from build123d import *

# Parameters (mm, degrees)
ESBO_O2_R                = 1.75
CORTE_EXTRUS_O1_DEPTH    = 6
ESBO_O3_R                = 4.25
CORTE_EXTRUS_O2_DEPTH    = 43.649736224
PADR_OCIRCULAR1_COUNT    = 4
CHANFRO1_SIZE            = 2
ESBO_O4_R                = 2
CORTE_EXTRUS_O3_DEPTH    = 46.639894829
PADR_OCIRCULAR2_COUNT    = 4
CHANFRO3_SIZE            = 2
RESSALTO_EXTRUS_O2_START = 2
ESBO_O5_R                = 12
ESBO_O5_R_2              = 1.75
RESSALTO_EXTRUS_O2_DEPTH = 2


with BuildPart() as part:
    # Esboço1 → Revolução1 (revolve)
    with BuildSketch(Plane.XY, mode=Mode.PRIVATE) as revolu_o1_sk:
        Polygon((0, 0), (0, 25), (27, 25), (27, 19), (12, 19), (12, 0), align=None)
    revolve(revolu_o1_sk.sketch.rotate(Axis((0, 0, 0), (0, 1, 0)), 90), axis=Axis((0, 0, 0), (0, 1, 0)))

    # Esboço2 → Corte-extrusão1 (cut)
    with BuildSketch(Plane.XZ):
        with Locations(Location((0, 7, 0), (0, 0, 270))):
            Circle(ESBO_O2_R)
    corte_extrus_o1 = extrude(amount=-CORTE_EXTRUS_O1_DEPTH, mode=Mode.SUBTRACT)

    # Esboço3 → Corte-extrusão2 (cut, through all)
    with BuildSketch(Plane.XZ.offset(-6)):
        with Locations(Location((0, 7, 0), (0, 0, 270))):
            Circle(ESBO_O3_R)
    corte_extrus_o2 = extrude(amount=-CORTE_EXTRUS_O2_DEPTH, mode=Mode.SUBTRACT)

    # PadrãoCircular1: Corte-extrusão1, Corte-extrusão2 ×4 about axis
    padr_ocircular1_axis = Axis((0, 0, 0), (0, 1, 0))
    add([corte_extrus_o1.rotate(padr_ocircular1_axis, i * 360 / PADR_OCIRCULAR1_COUNT) for i in range(1, PADR_OCIRCULAR1_COUNT)], mode=Mode.SUBTRACT)
    add([corte_extrus_o2.rotate(padr_ocircular1_axis, i * 360 / PADR_OCIRCULAR1_COUNT) for i in range(1, PADR_OCIRCULAR1_COUNT)], mode=Mode.SUBTRACT)

    # Chanfro1
    chanfro1_edges = [part.edges().sort_by_distance(p)[0] for p in [
        (0, 6, 8.75),
        (0, 6, -8.75),
        (8.75, 6, 0),
        (-8.75, 6, 0),
    ]]
    chamfer(chanfro1_edges, length=CHANFRO1_SIZE)

    # Esboço4 → Corte-extrusão3 (cut, through all)
    with BuildSketch(Plane(origin=(0, 25, 0), x_dir=(1, 0, 0), z_dir=(0, 1, 0))):
        with Locations(Location((-15.556349186, 15.556349186, 0), (0, 0, 270))):
            Circle(ESBO_O4_R)
    corte_extrus_o3 = extrude(amount=-CORTE_EXTRUS_O3_DEPTH, mode=Mode.SUBTRACT)

    # PadrãoCircular2: Corte-extrusão3 ×4 about axis
    padr_ocircular2_axis = Axis((0, 0, 0), (0, 1, 0))
    for i in range(1, PADR_OCIRCULAR2_COUNT):
        add(corte_extrus_o3.rotate(padr_ocircular2_axis, i * 360 / PADR_OCIRCULAR2_COUNT), mode=Mode.SUBTRACT)

    # Chanfro3
    chanfro3_edges = [part.edges().sort_by_distance(p)[0] for p in [
        (-15.556349186, 25, -17.556349186),
        (17.556349186, 25, -15.556349186),
        (15.556349186, 25, 17.556349186),
        (-17.556349186, 25, 15.556349186),
    ]]
    chamfer(chanfro3_edges, length=CHANFRO3_SIZE)

    # Esboço5 → Ressalto-extrusão2 (add)
    with BuildSketch(Plane.XZ.offset(RESSALTO_EXTRUS_O2_START)):
        with Locations(Location((0, 0, 0), (0, 0, 270))):
            Circle(ESBO_O5_R)
        with Locations(Location((-7, 0, 0), (0, 0, 270))):
            Circle(ESBO_O5_R_2, mode=Mode.SUBTRACT)
        with Locations(Location((0, -7, 0), (0, 0, 270))):
            Circle(ESBO_O5_R_2, mode=Mode.SUBTRACT)
        with Locations(Location((7, 0, 0), (0, 0, 270))):
            Circle(ESBO_O5_R_2, mode=Mode.SUBTRACT)
        with Locations(Location((0, 7, 0), (0, 0, 270))):
            Circle(ESBO_O5_R_2, mode=Mode.SUBTRACT)
    extrude(amount=-RESSALTO_EXTRUS_O2_DEPTH)


solid = part.part
Design review of the part built by this model. Coordinates are the model's own, in mm. A direction names the side the tool comes from. Round coordinates to 2 decimals unless told otherwise and drop trailing zeros. Order: outer loops, then holes, each group sorted by start corner. A loop starts at its lowest first (then second) coordinate and runs counter-clockwise, first axis right, second up. Notation, with made-up numbers: M 11.25,-10 L 26.25,-10 A17 cw 26.25,20 Z; hole C 58.5,67.25 d4. An arc over 180 degrees is marked long. Answer as CSV lines item,"result". Start each with the question number.
1) Wall thickness on line 1 along X through (y, z) = (18.5, 2); line 2 along X through (y, z) = (23, -2.5); line 3 along Y through (x, z) = (4, -14): over which ranges is each line inside the solid? List them lowest first. Write a range as [from, to].
2) Add section A-A (x = -7). Give the boundary of the cut face in (y, z).
3) Add section D-D (z = -7). Give the boundary of the cut face in (x, y).
4) Add section C-C (y = 16.75). Give the boundary of the cut face in (x, z), then the cut area to 3 significant figures.
5) Tool access review of faces 1 (the face through (17.51, 21.03, 15.99)), 2 (the face through (7, 6, 4)), 3 (the face through (6, 19, -12)): name each direction out of +Z, -Z, +X, -X, +Y, -Y from which nothing blocks a thin tool from reaching the whole face with its end or side.
6) Add section B-B (z = 0). Give the boundary of the cut face in (x, y), then the cut area to 3 significant figures.
7) The part is to be moulded in two halves that separate along Z. For faces 4 (the face through (26.36, 21.96, 5.85)), 5 (the face through (10.37, 15.37, 2.59)), 6 (the face through (0, -2, 0)), say which applies: +Z half, -Z half, draft (parallel to the pull), parting line (faces both ways), or undercut.
8) For pin 1 Ø4.5 at (x, z) = (7, 0) entering from +Y; pin 2 Ø7 at (x, z) = (0, 7) entering from +Y; pin 3 Ø2 at (x, z) = (-7, 0) entering from +Y; pin 4 Ø5 at (x, z) = (-15.56, 15.56) entering from -Y, all flat-tipped, find the tip position at first contact; note any pin that passes through.
Resolved:
1,line 1,"[-11.83, -10.75], [-3.25, 3.25], [10.75, 11.83]"
1,line 2,"[-26.88, -10.44], [-3.56, 3.56], [10.44, 26.88]"
1,line 3,"[19, 25]"
2,outline,"M -2,-9.75 L 19,-9.75 L 19,-26.08 L 25,-26.08 L 25,-4.25 L 6,-4.25 L 6,-3.75 L 4,-1.75 L -2,-1.75 Z; M -2,1.75 L 4,1.75 L 6,3.75 L 6,4.25 L 25,4.25 L 25,26.08 L 19,26.08 L 19,9.75 L -2,9.75 Z"
3,outline,"M -26.08,19 L -9.75,19 L -9.75,-2 L -1.75,-2 L -1.75,4 L -3.75,6 L -4.25,6 L -4.25,25 L -26.08,25 Z; M 1.75,-2 L 9.75,-2 L 9.75,19 L 26.08,19 L 26.08,25 L 4.25,25 L 4.25,6 L 3.75,6 L 1.75,4 Z"
4,outline,"C 0,0 d24; hole C -7,0 d8.5; hole C 0,-7 d8.5; hole C 0,7 d8.5; hole C 7,0 d8.5"
4,area,"225 mm^2"
5,face 1,"+Y, -Y"
5,face 2,"+Y"
5,face 3,"-Y"
6,outline,"M -27,19 L -12,19 L -12,-2 L -8.75,-2 L -8.75,4 L -10.75,6 L -11.25,6 L -11.25,25 L -27,25 Z; M -5.25,-2 L 5.25,-2 L 5.25,4 L 3.25,6 L 2.75,6 L 2.75,25 L -2.75,25 L -2.75,6 L -3.25,6 L -5.25,4 Z; M 8.75,-2 L 12,-2 L 12,19 L 27,19 L 27,25 L 11.25,25 L 11.25,6 L 10.75,6 L 8.75,4 Z"
6,area,"441 mm^2"
7,face 4,"parting line"
7,face 5,"undercut"
7,face 6,"draft"
8,pin 1,"y = 4.5"
8,pin 2,"y = 5.75"
8,pin 3,"through"
8,pin 4,"y = 19"
